Can you work these out from the model? Positions are in its coordinate system, mm. Round coordinates to 2 decimals unless told otherwise and drop trailing zeros. Write each loop counter-clockwise with the first axis right and the second up, starting at its lowest first coordinate (ties: lowest second). Pieces come first, ordered by that corner, then holes. Notation, with made-up numbers: (59.25, -36) -> (69.25, -36) arc R19 ccw to (69.25, -6) -> close; hole circle Ø9 at (18.5, -25.5). An arc over 180 degrees is marked (long way). Write item = value, one per line. Start each with the question number.
1) If I drill on line 1 (Z direction, x = -75, y = 0.2); line 2 (X direction, y = 0.75, z = 73.5), over which ranges is the centre line in solid material (lowest first)?
2) Imagine slicing it at B-B, the plane x = 75. Please give me the cut outline in (y, z).
3) Imagine slicing it at A-A, the plane z = -75. Please give me the cut outline in (x, y), then the cut area to 3 significant figures.
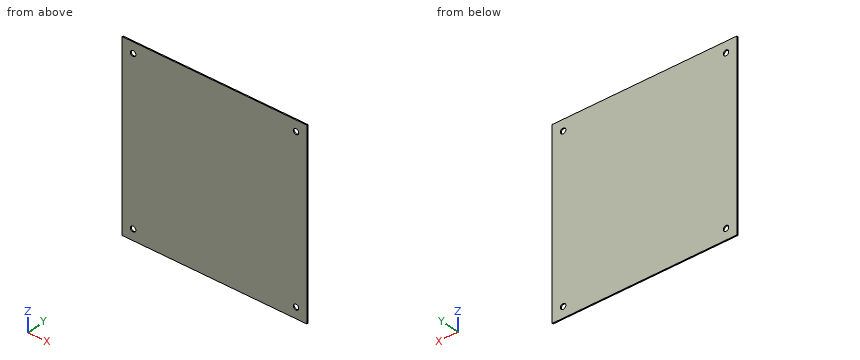
Solid Edge part; units mm, degrees
sketch "Sketch1" plane through (0, 0, 0) normal (0, -1, 0) x (1, 0, 0)
  line L0 (85, 85) -> (-85, 85)
  line L1 (-85, 85) -> (-85, -85)
  line L2 (-85, -85) -> (85, -85)
  line L3 (85, -85) -> (85, 85)
extrude "Protrusion1" add sketch "Sketch1" against normal blind 1
sketch "Sketch2" plane through (0, 0, 0) normal (0, -1, 0) x (1, 0, 0)
  circle A0 centre (-75, 75) radius 2.5
  circle A1 centre (75, 75) radius 2.5
  circle A2 centre (75, -75) radius 2.5
  circle A3 centre (-75, -75) radius 2.5
extrude "Cutout1" cut sketch "Sketch2" against normal through all
properties material "Aluminum, 1060"
Reported:
q1.line_1 = -85 to -77.5, -72.5 to 72.5, 77.5 to 85
q1.line_2 = -85 to -77, -73 to 73, 77 to 85
q2.outline = (0, -85) -> (1, -85) -> (1, -77.5) -> (0, -77.5) -> close; (0, -72.5) -> (1, -72.5) -> (1, 72.5) -> (0, 72.5) -> close; (0, 77.5) -> (1, 77.5) -> (1, 85) -> (0, 85) -> close
q3.outline = (-85, 0) -> (-77.5, 0) -> (-77.5, 1) -> (-85, 1) -> close; (-72.5, 0) -> (72.5, 0) -> (72.5, 1) -> (-72.5, 1) -> close; (77.5, 0) -> (85, 0) -> (85, 1) -> (77.5, 1) -> close
q3.area = 160 mm²
